Build history of the part. All positions in model axes, mm. Face numbers are marked on the shaded views. A direction names the side the tool comes from. Round coordinates to 2 decimals unless told otherwise and drop trailing zeros. Order: outer loops, then holes, each group sorted by start corner. A loop starts at its lowest first (then second) coordinate and runs counter-clockwise, first axis right, second up. Notation, with made-up numbers: (-12, -3.75) -> (16, -3.75) arc R22 cw to (16, 33.25) -> close; hole circle Ø5 at (-19.75, 48). An arc over 180 degrees is marked (long way). Write item = value, one per line.
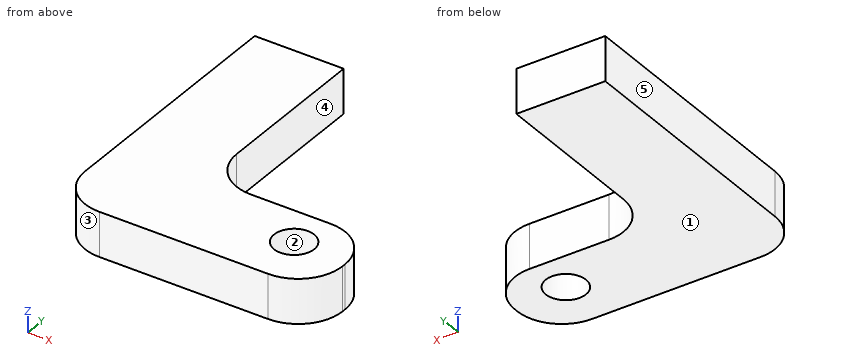
from build123d import *

# Parameters (mm, degrees)
SKETCH1_R           = 2.8702
BOSS_EXTRUDE1_DEPTH = 6.35
FILLET1_R           = 6.35


with BuildPart() as part:
    # Sketch1 → Boss-Extrude1 (new body)
    with BuildSketch(Plane.XY):
        Polygon((113.949884677, 0), (126.649884677, 0), (126.649884677, -6.35), (126.649884677, -28.855984936), (150.753776805, -28.855984936), (150.753776805, -42.040179878), (126.649884677, -42.040179878), (113.949884677, -42.040179878), (113.949884677, -6.35), align=None)
        with Locations((143.035641266, -34.539684717)):
            Circle(SKETCH1_R, mode=Mode.SUBTRACT)
    extrude(amount=BOSS_EXTRUDE1_DEPTH)

    # Fillet1
    fillet1_edges = [part.edges().sort_by_distance(p)[0] for p in [
        (126.649884677, -28.855984936, 3.175),
        (150.753776805, -28.855984936, 3.175),
        (150.753776805, -42.040179878, 3.175),
        (113.949884677, -42.040179878, 3.175),
    ]]
    fillet(fillet1_edges, radius=FILLET1_R)


solid = part.part
Q1. Mould opens along Y. For the marked faces 1, 2 and 3 say: released by +Y, released by -Y, zero draft, split by the parting line, or undercut.
Check values:
face_1 = zero draft
face_2 = undercut
face_3 = released by -Y
Q2. Which spindle directions (+Z, -Z, +X, -X, +Y, -Y) get a long thin tool onto all of the face, cutting with end or side? Do the marked faces 4 and 5. Say none if no direction does.
Check values:
face_4 = +Z, -Z, +X, +Y
face_5 = +Z, -Z, -X, +Y, -Y
Q3. Cut at A-A, the plane z = 2. List the corners of the cut face in (x, y), and give its area (3 significant figures).
Check values:
outline = (113.95, -35.69) arc R6.35 ccw to (120.3, -42.04) -> (144.4, -42.04) arc R6.35 ccw to (150.75, -35.69) -> (150.75, -35.21) arc R6.35 ccw to (144.4, -28.86) -> (133, -28.86) arc R6.35 cw to (126.65, -22.51) -> (126.65, 0) -> (113.95, 0) -> close; hole circle Ø5.74 at (143.04, -34.54)
area = 809 mm²
Q4. Cut at B-B, the plane y = -12. List the corners of the cut face in (x, z).
Check values:
outline = (113.95, 0) -> (126.65, 0) -> (126.65, 6.35) -> (113.95, 6.35) -> close
Q5. Cut at C-C, the plane x = 138.5. List the corners of the cut face in (y, z), and give its area (3 significant figures).
Check values:
outline = (-42.04, 0) -> (-28.86, 0) -> (-28.86, 6.35) -> (-42.04, 6.35) -> close
area = 83.7 mm²
Q6. Probe probe 1 along Y at (x, z) = (143, 4); probe 2 along Y at (x, z) = (120, 4); probe 3 along Y at (x, z) = (135, 2.75). List the from-to ranges inside material, lowest first.
Check values:
probe_1 = -42.04 to -37.41, -31.67 to -28.86
probe_2 = -42.03 to 0
probe_3 = -42.04 to -28.86
Q7. Flat gauge pins, fed straight in: pin 1 (3 mm diameter, centred on x = 147, z = 2.5, fed in from +Y); pin 2 (2 mm diameter, centred on y = -20, z = 3, fed in from +X). Where does each tip first touch, or does it go through?
Check values:
pin_1 = -28.95
pin_2 = 126.65
